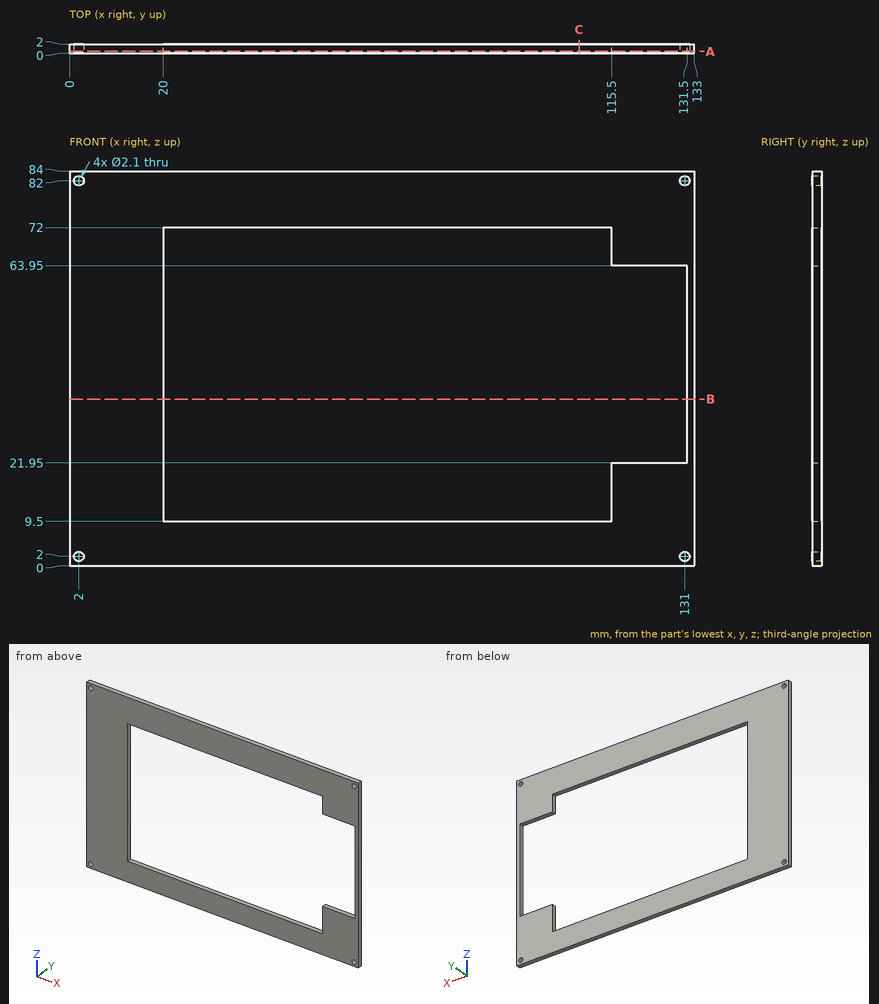
Could you check a few things on this drawing? It's one solid part, dimensions in mm from its lowest x, y, z. Coordinates: 2 decimals unless noted, no trailing zeros. Loops run counter-clockwise (first coordinate to the right, second up) from the corner with the lowest first, then second, coordinate; pieces in that order, holes last. Notation, with made-up numbers: (40, -37) - (45, -37) arc R19 cw to (45, -8) - close; hole circle Ø3 at (-24, 26.5). An arc over 180 degrees is marked (long way). Answer as a JSON object with one key per item and string values. Group by question number.
Item 1: If we section it at B-B (z = 35.5): List the corners of the cut face in (x, y) for me.
Item 2: If we section it at C-C (x = 108.5): List the corners of the cut face in (y, z) for me.
Item 3: If we section it at A-A (y = 0.45): List the corners of the cut face in (x, z) for me, plus the area to 3 significant figures.
Item 4: If I drill on L1, parallel to Z at x = 131, y = 0.95; L2, parallel to X at y = 1, z = 2; L3, parallel to Z at x = 84.5, y = 0.9, over which ranges is the centre line in solid material (lowest first)? Write a range as from..to.
Item 5: For pin 1 (1 mm diameter, centred on x = 22, z = 49, fed in from +Y), with a flat end and sliding along its axis, tell me the tip position at first contact or that it passes through.
Returned:
{
 "1": {"outline": "(0, 0) - (20, 0) - (20, 2) - (0, 2) - close; (131.5, 0) - (133, 0) - (133, 2) - (131.5, 2) - close"},
 "2": {"outline": "(0, 0) - (2, 0) - (2, 9.5) - (0, 9.5) - close; (0, 72) - (2, 72) - (2, 84) - (0, 84) - close"},
 "3": {"outline": "(0, 0) - (133, 0) - (133, 84) - (0, 84) - close; hole circle Ø2.1 at (2, 2); hole circle Ø2.1 at (2, 82); hole (20, 9.5) - (115.5, 9.5) - (115.5, 21.95) - (131.5, 21.95) - (131.5, 63.95) - (115.5, 63.95) - (115.5, 72) - (20, 72) - close; hole circle Ø2.1 at (131, 2); hole circle Ø2.1 at (131, 82)", "area": "4,520 mm²"},
 "4": {"L1": "z = 0..0.95, 3.05..21.95, 63.95..80.95, 83.05..84", "L2": "x = 0..0.95, 3.05..129.95, 132.05..133", "L3": "z = 0..9.5, 72..84"},
 "5": {"pin 1": "passes through"}
}
